Could you check a few things on this drawing? It's one solid part, dimensions in mm from its lowest x, y, z. A direction names the side the tool comes from. Round coordinates to 2 decimals unless told otherwise and drop trailing zeros. Write each loop counter-clockwise with the first axis right and the second up, starting at its lowest first coordinate (ties: lowest second). Pieces come first, ordered by that corner, then holes. Notation, with made-up numbers: (68.5, -15.5) - (123.5, -15.5) arc R19 cw to (123.5, 19.5) - close; hole circle Ø9 at (-17.75, -22.5). An arc over 180 degrees is marked (long way). Use one line per item in the form item = value. Start each with the question number.
1. Which directions (+Z, -Z, +X, -X, +Y, -Y) give clear straight access to the entire face, cutting with the end or side of a thin tool? Please do the marked faces 4 and 5.
2. Will these pins go through, and if not, where does the flat tip stop? pin 1 (4 mm diameter, centred on x = 12.5, y = 6, fed in from +Z); pin 2 (1.8 mm diameter, centred on x = 10, y = 10, fed in from +Z); pin 3 (5 mm diameter, centred on y = 13.5, z = 13.5, fed in from +X); pin 4 (2 mm diameter, centred on x = 34, y = 11.5, fed in from +Z).
3. I want a section at D-D, the plane x = 50. List the corners of the cut face in (y, z) for me.
4. I want a section at B-B, the plane x = 30. List the corners of the cut face in (y, z) for me, plus the area to 3 significant figures.
5. We'd pull the mould along X, two halves only. Please class the marked faces 1, 2 and 3: +X half, -X half, draft (parallel to the pull), parting line (faces both ways), or undercut.
6. If I drill on line 1 along Y through (x, z) = (50, 6); line 2 along X through (y, z) = (3.75, 9.75); line 3 along Z through (x, y) = (19.5, 4.75), over which ranges is the centre line in solid material (lowest first)?
7. I want a section at C-C, the plane y = 3.5. List the corners of the cut face in (x, z) for me (1 decimal).
8. I want a section at A-A, the plane y = 10. List the corners of the cut face in (x, z) for me (1 decimal).
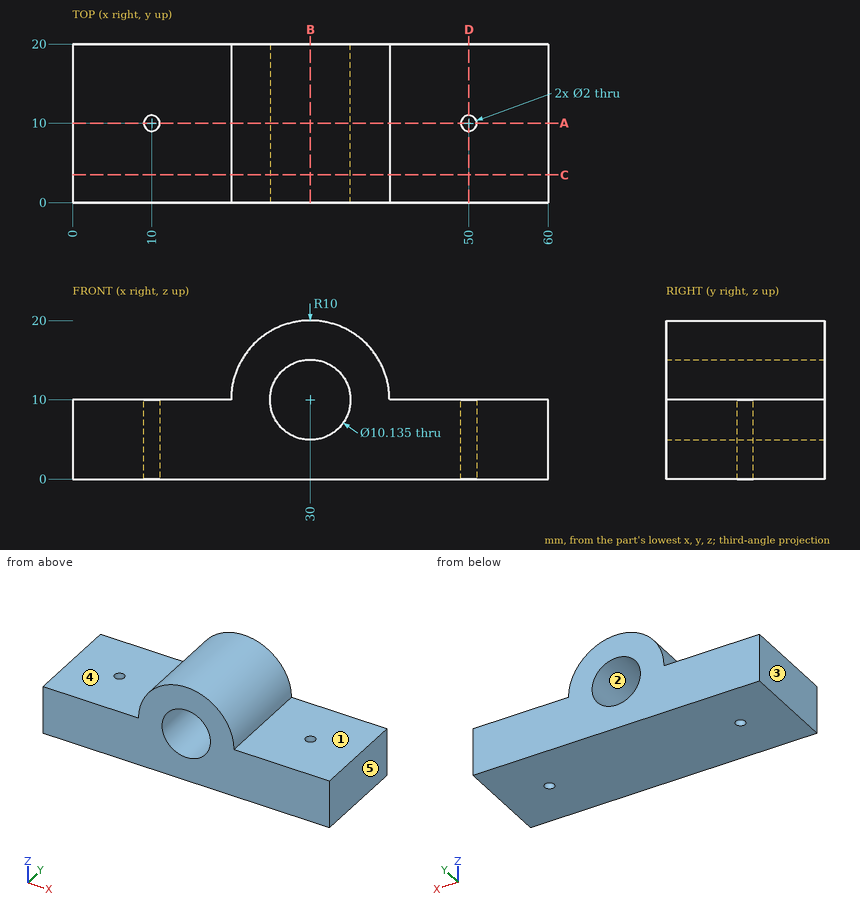
Model answer:
q1.face_4 = +Z, -X, +Y, -Y
q1.face_5 = +Z, -Z, +X, +Y, -Y
q2.pin_1 = 10
q2.pin_2 = through
q2.pin_3 = 39.95
q2.pin_4 = 19.54
q3.outline = (0, 0) - (9, 0) - (9, 10) - (0, 10) - close; (11, 0) - (20, 0) - (20, 10) - (11, 10) - close
q4.outline = (0, 0) - (20, 0) - (20, 4.93) - (0, 4.93) - close; (0, 15.07) - (20, 15.07) - (20, 20) - (0, 20) - close
q4.area = 197 mm2
q5.face_1 = draft
q5.face_2 = undercut
q5.face_3 = -X half
q6.line_1 = 0 to 9, 11 to 20
q6.line_2 = 0 to 24.94, 35.06 to 60
q6.line_3 = 0 to 10
q7.outline = (0, 0) - (60, 0) - (60, 10) - (40, 10) arc R10 ccw to (20, 10) - (0, 10) - close; hole circle Ø10.1 at (30, 10)
q8.outline = (0, 0) - (9, 0) - (9, 10) - (0, 10) - close; (11, 0) - (49, 0) - (49, 10) - (40, 10) arc R10 ccw to (20, 10) - (11, 10) - close; (51, 0) - (60, 0) - (60, 10) - (51, 10) - close; hole circle Ø10.1 at (30, 10)
